Could you check a few things on this model? Use its own coordinates, in mm. Coordinates: 2 decimals unless noted, no trailing zeros. Loops run counter-clockwise (first coordinate to the right, second up) from the corner with the lowest first, then second, coordinate; pieces in that order, holes last. Notation, with made-up numbers: M -34.5,41.25 L 4.5,41.25 A13 ccw 4.5,65.25 Z; hole C 12.25,85.25 d7. An arc over 180 degrees is marked long. Return JSON: item names as keys, results as strings. Group by question number.
Autodesk Inventor part; units mm, degrees
ref_plane "Work Plane32" through (254, 330.2, 0) normal (0, 0, -1) x (-1, 0, 0)
ref_plane "Work Plane28" through (254, 330.2, -6.35) normal (0, 0, -1) x (-1, 0, 0)
ref_plane "YZ Plane" through (0, 0, 0) normal (1, 0, 0) x (0, 1, 0)
ref_plane "Work Plane32" through (254, 330.2, 0) normal (0, 0, -1) x (-1, 0, 0)
sketch "Sketch36" plane through (254, 330.2, 0) normal (0, 0, -1) x (-1, 0, 0)
  line L0 (254, -363.855) -> (254, -196.85)
  line L1 (0, 0) -> (0, -114.3)
  line L2 (254, -363.855) -> (0, -363.855)
  line L3 (0, -363.855) -> (0, 0)
  line L4 (0, 0) -> (254, 0)
  line L5 (254, 0) -> (254, -363.855)
  line L6 (342.9, -196.85) -> (342.9, -114.3)
  line L7 (342.9, -196.85) -> (254, -196.85)
  line L8 (254, -196.85) -> (254, -114.3)
  line L9 (254, -114.3) -> (342.9, -114.3)
  line L10 (342.9, -114.3) -> (342.9, -196.85)
  line L11 (-31.75, -363.855) -> (254, -363.855)
  line L12 (0, -314.325) -> (0, -196.85)
  line L13 (-31.75, -363.855) -> (0, -363.855)
  line L14 (0, -363.855) -> (0, -314.325)
  line L15 (0, -314.325) -> (-31.75, -314.325)
  line L16 (-31.75, -314.325) -> (-31.75, -363.855)
  line L17 (0, -196.85) -> (-88.9, -196.85)
  line L18 (-88.9, -196.85) -> (-88.9, -114.3)
  line L19 (-88.9, -114.3) -> (0, -114.3)
  line L20 (0, -114.3) -> (0, -196.85)
  dimension "d412" = 82.55
  dimension "d413" = 254
  dimension "d414" = 31.75
extrude "Extrusion20" add sketch "Sketch36" along normal blind 6.35
ref_plane "Work Plane28" through (254, 330.2, -6.35) normal (0, 0, -1) x (-1, 0, 0)
sketch "Sketch39" plane through (254, 330.2, -6.35) normal (0, 0, -1) x (-1, 0, 0)
  line L0 (0, -196.85) -> (0, -314.325)
  line L1 (0, -196.85) -> (5.08, -196.85)
  line L2 (5.08, -196.85) -> (5.08, -314.325)
  line L3 (5.08, -314.325) -> (0, -314.325)
  line L4 (0, -314.325) -> (0, -196.85)
  line L5 (254, -363.855) -> (254, -196.85)
  line L6 (-31.75, -363.855) -> (254, -363.855)
  line L7 (254, -196.85) -> (248.92, -196.85)
  line L8 (248.92, -196.85) -> (248.92, -363.855)
  line L9 (248.92, -363.855) -> (254, -363.855)
  line L10 (254, -363.855) -> (254, -196.85)
  line L11 (0, -114.3) -> (-88.9, -114.3)
  line L12 (254, 0) -> (0, 0)
  line L13 (0, -114.3) -> (5.08, -114.3)
  line L14 (5.08, -114.3) -> (5.08, 0)
  line L15 (5.08, 0) -> (0, 0)
  line L16 (0, 0) -> (0, -114.3)
  line L17 (254, 0) -> (248.92, 0)
  line L18 (248.92, 0) -> (248.92, -114.3)
  line L19 (248.92, -114.3) -> (254, -114.3)
  line L20 (254, -114.3) -> (254, 0)
  point P0 (254, -330.2)
  dimension "d415" = 5.08
  dimension "d416" = 5.08
  dimension "d417" = 5.08
extrude "Extrusion22" cut sketch "Sketch39" against normal blind 6.35
sketch "Sketch41" plane through (254, 330.2, 0) normal (0, 0, 1) x (1, 0, 0)
  line L0 (-5.08, -314.325) -> (31.75, -314.325)
  line L1 (31.75, -363.855) -> (-248.92, -363.855)
  line L2 (31.75, -314.325) -> (-5.08, -314.325)
  line L3 (-5.08, -314.325) -> (-5.08, -363.855)
  line L4 (-5.08, -363.855) -> (31.75, -363.855)
  line L5 (31.75, -363.855) -> (31.75, -314.325)
  point P0 (-254, -330.2)
  dimension "d448" = 36.83
extrude "Extrusion24" cut sketch "Sketch41" against normal blind 6.35
properties part number "20Gen2PlatePart"
(1) Imagine slicing it at A-A, the plane z = -1.25. Write out the boundary of the cut face in (x, y) (3 decimals), then the cut area to 3 significant figures.
(2) Imagine slicing it at C-C, the plane y = 91. Write out the boundary of the cut face in (x, z), then the cut area to 3 significant figures.
(3) If I drill on L1, parallel to X at y = 80, z = -0.75; L2, parallel to Y at x = 292, z = -1.75, over which ranges is the centre line in solid material (lowest first)? Write a range as [from, to].
(4) Will these pins go through, and if not, where does the flat tip stop? P1, Ø1.9, axis at y = 248.5, z = -2, coming from the -X side; P2, Ø1.9, axis at x = 277, z = -3.5, coming from the -Y side; P3, Ø3, axis at y = 31, z = -2.5, coming from the +X side.
(5) Imagine slicing it at B-B, the plane x = -51. Write out the boundary of the cut face in (y, z), then the cut area to 3 significant figures.
Checks:
{
 "1": {"outline": "M -88.9,133.35 L 5.08,133.35 L 5.08,-33.655 L 248.92,-33.655 L 248.92,133.35 L 342.9,133.35 L 342.9,215.9 L 248.92,215.9 L 248.92,330.2 L 5.08,330.2 L 5.08,215.9 L -88.9,215.9 Z", "area": "104,000 mm²"},
 "2": {"outline": "M 5.08,-6.35 L 248.92,-6.35 L 248.92,0 L 5.08,0 Z", "area": "1,550 mm²"},
 "3": {"L1": "[5.08, 248.92]", "L2": "[133.35, 215.9]"},
 "4": {"P1": "x = 5.08", "P2": "y = 133.35", "P3": "x = 248.92"},
 "5": {"outline": "M 133.35,-6.35 L 215.9,-6.35 L 215.9,0 L 133.35,0 Z", "area": "524 mm²"}
}
